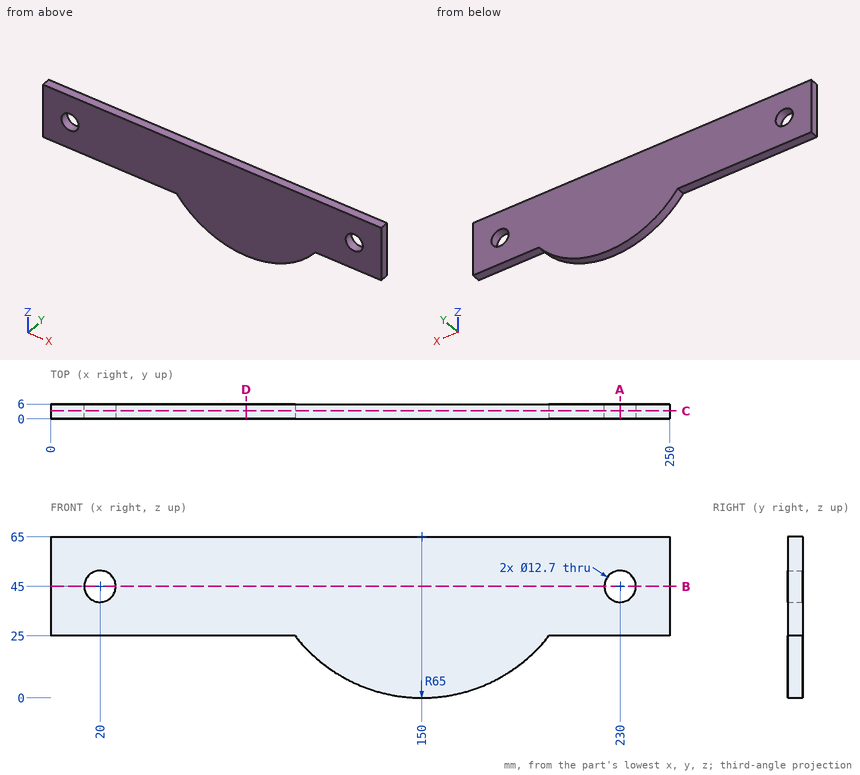
Geometry check sheet. Reference: drawing and pictorial views, mm from the part's lowest x, y, z. Coordinates: 2 decimals unless noted, no trailing zeros. Write each loop counter-clockwise with the first axis right and the second up, starting at its lowest first coordinate (ties: lowest second). Pieces come first, ordered by that corner, then holes. Notation, with made-up numbers: (8.5, 40) -> (39.5, 40) arc R28 ccw to (39.5, 58) -> close; hole circle Ø11 at (18, 9). An arc over 180 degrees is marked (long way). One line per question, with ' | ' between items.
1. Thickness scan on probe 1 along X at (y, z) = (1.1, 45.5); probe 2 along Z at (x, y) = (230, 3.4); probe 3 along X at (y, z) = (2.9, 41.5). Record the ranges inside material, lowest first. Write a range as from..to.
Answers:
probe 1: x = 0..13.67, 26.33..223.67, 236.33..250 | probe 2: z = 25..38.65, 51.35..65 | probe 3: x = 0..14.7, 25.3..224.7, 235.3..250
2. Cross-section at D-D on x = 79. Record the cut outline in (y, z).
Answers:
outline: (0, 25) -> (6, 25) -> (6, 65) -> (0, 65) -> close
3. Cross-section at A-A on x = 230. Record the cut outline in (y, z), and give its area (3 significant figures).
Answers:
outline: (0, 25) -> (6, 25) -> (6, 38.65) -> (0, 38.65) -> close; (0, 51.35) -> (6, 51.35) -> (6, 65) -> (0, 65) -> close | area: 164 mm²
4. Cross-section at C-C on y = 3.2. Record the cut outline in (x, z), and give its area (3 significant figures).
Answers:
outline: (0, 25) -> (98.77, 25) arc R65 ccw to (201.23, 25) -> (250, 25) -> (250, 65) -> (0, 65) -> close; hole circle Ø12.7 at (20, 45); hole circle Ø12.7 at (230, 45) | area: 11,500 mm²
5. Depth check by flat-ended pin: pin 1 Ø1.5 at (y, z) = (4, 14) entering from -X. Enter the tip coordinate at first touch or a pass-through.
Answers:
pin 1: stops at x = 108.77
6. Cross-section at B-B on z = 45. Record the cut outline in (x, y), and give its area (3 significant figures).
Answers:
outline: (0, 0) -> (13.65, 0) -> (13.65, 6) -> (0, 6) -> close; (26.35, 0) -> (223.65, 0) -> (223.65, 6) -> (26.35, 6) -> close; (236.35, 0) -> (250, 0) -> (250, 6) -> (236.35, 6) -> close | area: 1,350 mm²
